Autodesk Inventor part; units mm, degrees
ref_plane "YZ Plane" through (0, 0, 0) normal (1, 0, 0) x (0, 1, 0)
ref_plane "XZ Plane" through (0, 0, 0) normal (0, 1, 0) x (-1, 0, 0)
ref_plane "XY Plane" through (0, 0, 0) normal (0, 0, 1) x (1, 0, 0)
sketch "Sketch1" plane through (0, 0, 0) normal (1, 0, 0) x (0, 1, 0)
  line L0 (0, 0) -> (25.4, 0)
  line L1 (25.4, 0) -> (25.4, 76.2)
  line L2 (25.4, 76.2) -> (0, 76.2)
  line L3 (0, 76.2) -> (0, 0)
  dimension "d2" = 25.4
  dimension "d3" = 76.2
extrude "Extrusion1" add sketch "Sketch1" along normal blind 25.4
sketch "Sketch2" plane through (25.4, 0, 0) normal (1, 0, 0) x (0, 0, -1)
  circle A0 centre (-717.1181, 162.0804) radius 50.8
  circle A1 centre (-57.15, 12.7) radius 5.08
  circle A2 centre (-38.1, 12.7) radius 5.08
  circle A3 centre (-19.05, 12.7) radius 5.08
  line L0 (0, 25.4) -> (-76.2, 25.4)
  line L1 (-76.2, 0) -> (0, 0)
  line L2 (-76.2, 25.4) -> (-76.2, 0)
  line L3 (0, 0) -> (0, 25.4)
  dimension "d6" = 101.6
  dimension "d15" = 10.16
  dimension "d16" = 10.16
  dimension "d17" = 10.16
  dimension "d18" = 25.4
  dimension "d19" = 12.7
  dimension "d21" = 76.2
  dimension "d22" = 38.1
  dimension "d23" = 19.05
  dimension "d24" = 25.4
  dimension "d26" = 19.05
  dimension "d27" = 12.7
extrude "Extrusion2" add sketch "Sketch2" along normal blind 50.8 contours A1 | A2 | A3
equation "\"d16\" = d15"
equation "\"d17\" = d15"
equation "\"d19\" = 0.5 * d18"
equation "\"d22\" = 0.5 * d21"
equation "\"d23\" = 0.5 * d22"
equation "\"d26\" = d23"
equation "\"d27\" = d19"
Verification items for the finished model (mm, model axes). A direction names the side the tool comes from. Coordinates: 2 decimals unless noted, no trailing zeros. Loops run counter-clockwise (first coordinate to the right, second up) from the corner with the lowest first, then second, coordinate; pieces in that order, holes last. Notation, with made-up numbers: (-34.75, 0.25) - (-23.75, 0.25) arc R31 cw to (-23.75, 24.25) - close; hole circle Ø8 at (-18, -8). An arc over 180 degrees is marked (long way). Put each result on its own line as item: value.
Item 1: Section check A-A (z = 57.15). Enter the section's corners in (x, y), then the cut area to 3 significant figures.
Conclusion:
outline: (0, 0) - (25.4, 0) - (25.4, 7.62) - (76.2, 7.62) - (76.2, 17.78) - (25.4, 17.78) - (25.4, 25.4) - (0, 25.4) - close
area: 1,160 mm2
Item 2: Gauge pin test, flat ends, axial feed: pin 1 Ø2 at (y, z) = (4, 62.5) entering from +X; pin 2 Ø2 at (x, z) = (63, 52) entering from +Y. Record the tip position at first contact, or that the pin passes through.
Conclusion:
pin 1: stops at x = 25.4
pin 2: stops at y = 15.63
Item 3: Set-up check for faces 1 (the face through (25.4, 18, 39)), 2 (the face through (0, 13, 39)): record each of +Z, -Z, +X, -X, +Y, -Y from which the full face is reachable in a straight line by a thin tool's end or side.
Conclusion:
face 1: +X
face 2: +Z, -Z, -X, +Y, -Y
Item 4: Scan lines: line 1 along Z through (x, y) = (52.5, 14); line 2 along Z through (x, y) = (53, 15.5); line 3 along X through (y, z) = (17.75, 6). Record each from-to range of solid material in increasing order.
Conclusion:
line 1: z = 14.14 to 23.96, 33.19 to 43.01, 52.24 to 62.06
line 2: z = 14.81 to 23.29, 33.86 to 42.34, 52.91 to 61.39
line 3: x = 0 to 25.4
Item 5: Section check C-C (x = 46). Enter the section's corners in (y, z), then the cut area to 3 significant figures.
Conclusion:
outline: circle Ø10.16 at (12.7, 19.05); circle Ø10.16 at (12.7, 38.1); circle Ø10.16 at (12.7, 57.15)
area: 243 mm2
Item 6: Draft check along Z on faces 3 (the face through (50.44, 17.66, 39.2)), 4 (the face through (13, 25.4, 38)), 5 (the face through (13, 13, 0)). Enter one of: pulls with the +Z half, pulls with the -Z half, needs draft (parallel to the pull), parting line crosses it, or undercut.
Conclusion:
face 3: undercut
face 4: needs draft
face 5: pulls with the -Z half
Item 7: Section check D-D (z = 46.5). Enter the section's corners in (x, y), then the cut area to 3 significant figures.
Conclusion:
outline: (0, 0) - (25.4, 0) - (25.4, 25.4) - (0, 25.4) - close
area: 645 mm2
Item 8: Section check B-B (y = 12.7). Enter the section's corners in (x, z), then the cut area to 3 significant figures.
Conclusion:
outline: (0, 0) - (25.4, 0) - (25.4, 13.97) - (76.2, 13.97) - (76.2, 24.13) - (25.4, 24.13) - (25.4, 33.02) - (76.2, 33.02) - (76.2, 43.18) - (25.4, 43.18) - (25.4, 52.07) - (76.2, 52.07) - (76.2, 62.23) - (25.4, 62.23) - (25.4, 76.2) - (0, 76.2) - close
area: 3,480 mm2
